Input: part model. Units: mm. Frame: model coordinates. A direction names the side the tool comes from. Give positions to 0.01 mm unless a question says otherwise; leave off trailing zeros. Loops run counter-clockwise (first coordinate to the right, second up) from the corner with the lowest first, then second, coordinate; pieces in that order, holes last. Notation, with made-up numbers: (-34, -29.5) - (-20, -29.5) arc R14 ccw to (-20, -5.5) - close; hole circle Ø9 at (-22, -9.75). An arc over 180 degrees is marked (long way). Answer as a JSON object with one key per item and string values. Group by question number.
(1) Pin query (flat end, axial travel): P1, Ø3, axis at y = -7, z = 6.5, coming from the +X side; P2, Ø3, axis at y = -3, z = 6.5, coming from the -X side; P3, Ø1.8, axis at y = -3.26, z = 6, coming from the +X side; P4, Ø3, axis at x = -1.5, y = -1, coming from the +Z side. Return the tip coordinate at first contact, or that it passes through.
(2) Section query C-C (x = 5). Return loops of the section in (y, z), plus the area to 3 significant figures.
(3) Mould query, pull axis Y, two halves, no side actions, for faces 1 (the flat face through (-7.927, -1, -1)), 2 (the flat face through (9, -6.26, 6)), 3 (the flat face through (1, -3.06, -5)). Classes: +Y half, -Y half, draft (parallel to the pull), parting line (faces both ways), or undercut.
(4) Access query for faces 4 (the flat face through (1, -3.46, -5)), 5 (the flat face through (-6, -0.26, 6)), 6 (the flat face through (-6, -6.26, 6)), 7 (the flat face through (-7.19, -5.59, 7.66)), 8 (the flat face through (1, -3, 0)). Directions: +Z, -Z, +X, -X, +Y, -Y. A direction counts if a zero-diameter tool reaches every point of the face in a straight line with its end or side. Return the directions, or none.
(5) Section query A-A (z = -4.5). Return loops of the section in (x, y), plus the area to 3 significant figures.
(6) Material intervals for L1, parallel to Z at x = -2.25, y = -3; L2, parallel to Y at x = 4.75, z = -5.25; L3, parallel to Y at x = 4, z = -2.5, sorted ascending.
(7) Section query B-B (y = -2.75). Return loops of the section in (x, z), plus the area to 3 significant figures.
(8) Section query D-D (z = 6). Return loops of the section in (x, y).
```python
from build123d import *

# Parameters (mm, degrees)
CROQUIS1_W              = 18
CROQUIS1_H              = 10
SALIENTE_EXTRUIR1_DEPTH = 3
CROQUIS2_W              = 6.078202003
CROQUIS2_H              = 6
CROQUIS2_R              = 1.5
SALIENTE_EXTRUIR2_DEPTH = 3
SALIENTE_EXTRUIR3_START = -18
CROQUIS2_2_W            = 6.078202003
CROQUIS2_2_H            = 6
CROQUIS2_2_R            = 1.5
SALIENTE_EXTRUIR3_DEPTH = 4
CORTAR_EXTRUIR1_DEPTH   = 1.5
SALIENTE_EXTRUIR4_DEPTH = 18


with BuildPart() as part:
    # Croquis1 → Saliente-Extruir1 (new body)
    with BuildSketch(Plane.XY):
        with Locations((1.07264213, -3.260188088)):
            Rectangle(CROQUIS1_W, CROQUIS1_H)
    extrude(amount=SALIENTE_EXTRUIR1_DEPTH)

    # Croquis2 → Saliente-Extruir2 (add)
    with BuildSketch(Plane(origin=(10.07264213, 0, 0), x_dir=(0, 0, -1), z_dir=(1, 0, 0))):
        with Locations((-6.039101002, -3.260188088)):
            Rectangle(CROQUIS2_W, CROQUIS2_H)
        with Locations((-5.99926787, -3.260188088)):
            Circle(CROQUIS2_R, mode=Mode.SUBTRACT)
    extrude(amount=-SALIENTE_EXTRUIR2_DEPTH)

    # Croquis2<2> → Saliente-Extruir3 (add)
    with BuildSketch(Plane(origin=(10.07264213, 0, 0), x_dir=(0, 0, -1), z_dir=(1, 0, 0)).offset(SALIENTE_EXTRUIR3_START)):
        with Locations((-6.039101002, -3.260188088)):
            Rectangle(CROQUIS2_2_W, CROQUIS2_2_H)
        with Locations((-5.99926787, -3.260188088)):
            Circle(CROQUIS2_2_R, mode=Mode.SUBTRACT)
    extrude(amount=SALIENTE_EXTRUIR3_DEPTH)

    # Croquis3 → Cortar-Extruir1 (cut)
    with BuildSketch(Plane.ZY.offset(7.92735787)):
        Polygon((5.99926787, -6.551084622), (8.84926787, -4.905636355), (8.84926787, -1.614739821), (5.99926787, 0.030708447), (3.14926787, -1.614739821), (3.14926787, -4.905636355), align=None)
    extrude(amount=-CORTAR_EXTRUIR1_DEPTH, mode=Mode.SUBTRACT)

    # Croquis4 → Saliente-Extruir4 (add)
    with BuildSketch(Plane(origin=(10.07264213, 0, 0), x_dir=(0, 0, -1), z_dir=(1, 0, 0))):
        Polygon((4, -1.260188088), (4, -3.060188088), (6, -3.060188088), (6, -1.260188088), (6, 1.739811912), (0, 1.739811912), (0, -1.260188088), align=None)
        Polygon((0, -8.260188088), (6, -8.260188088), (6, -5.260188088), (6, -3.460188088), (4, -3.460188088), (4, -5.260188088), (0, -5.260188088), align=None)
    extrude(amount=-SALIENTE_EXTRUIR4_DEPTH)


solid = part.part
```
Recorded:
{
 "1": {"P1": "stops at x = 10.07", "P2": "stops at x = -6.43", "P3": "passes through", "P4": "stops at z = 3"},
 "2": {"outline": "(-8.26, -6) - (-3.46, -6) - (-3.46, -4) - (-5.26, -4) - (-5.26, 0) - (-1.26, 0) - (-1.26, -4) - (-3.06, -4) - (-3.06, -6) - (1.74, -6) - (1.74, 3) - (-8.26, 3) - close", "area": "73.2 mm^2"},
 "3": {"face 1": "draft", "face 2": "-Y half", "face 3": "undercut"},
 "4": {"face 4": "-Z, +X, -X", "face 5": "+Z, +X, -X, +Y", "face 6": "+Z, +X, -X, -Y", "face 7": "-X", "face 8": "+X, -X"},
 "5": {"outline": "(-7.93, -8.26) - (10.07, -8.26) - (10.07, -3.46) - (-7.93, -3.46) - close; (-7.93, -3.06) - (10.07, -3.06) - (10.07, 1.74) - (-7.93, 1.74) - close", "area": "173 mm^2"},
 "6": {"L1": "z = -6 to -4, 0 to 3", "L2": "y = -8.26 to -3.46, -3.06 to 1.74", "L3": "y = -8.26 to -5.26, -1.26 to 1.74"},
 "7": {"outline": "(-7.93, -6) - (10.07, -6) - (10.07, -4) - (-7.93, -4) - close; (-7.93, 0) - (10.07, 0) - (10.07, 4.59) - (7.07, 4.59) - (7.07, 3) - (-3.93, 3) - (-3.93, 4.59) - (-6.43, 4.59) - (-6.43, 3.15) - (-7.93, 3.15) - close; (-7.93, 8.85) - (-6.43, 8.85) - (-6.43, 7.41) - (-3.93, 7.41) - (-3.93, 9.08) - (-7.93, 9.08) - close; (7.07, 7.41) - (10.07, 7.41) - (10.07, 9.08) - (7.07, 9.08) - close", "area": "108 mm^2"},
 "8": {"outline": "(-6.43, -6.26) - (-3.93, -6.26) - (-3.93, -4.76) - (-6.43, -4.76) - close; (-6.43, -1.76) - (-3.93, -1.76) - (-3.93, -0.26) - (-6.43, -0.26) - close; (7.07, -6.26) - (10.07, -6.26) - (10.07, -4.76) - (7.07, -4.76) - close; (7.07, -1.76) - (10.07, -1.76) - (10.07, -0.26) - (7.07, -0.26) - close"}
}
